```python
from build123d import *

# Parameters (mm, degrees)
SKETCH1_R           = 300
BOSS_EXTRUDE1_DEPTH = 8
SKETCH2_R           = 8
CUT_EXTRUDE1_DEPTH  = 425.339486732


with BuildPart() as part:
    # Sketch1 → Boss-Extrude1 (new body)
    with BuildSketch(Plane(origin=(0, 0, 0), x_dir=(1, 0, 0), z_dir=(0, 1, 0))):
        with Locations(Location((0, 0, 0), (0, 0, 270))):
            Circle(SKETCH1_R)
    extrude(amount=BOSS_EXTRUDE1_DEPTH)

    # Sketch2 → Cut-Extrude1 (cut, through all)
    with BuildSketch(Plane.XZ):
        with Locations(Location((0, 60, 0), (0, 0, 270))):
            Circle(SKETCH2_R)
        with Locations(Location((30, 51.961524227, 0), (0, 0, 270))):
            Circle(SKETCH2_R)
        with Locations(Location((51.961524227, 30, 0), (0, 0, 270))):
            Circle(SKETCH2_R)
        with Locations(Location((60, 0, 0), (0, 0, 270))):
            Circle(SKETCH2_R)
        with Locations(Location((51.961524227, -30, 0), (0, 0, 270))):
            Circle(SKETCH2_R)
        with Locations(Location((30, -51.961524227, 0), (0, 0, 270))):
            Circle(SKETCH2_R)
        with Locations(Location((0, -60, 0), (0, 0, 270))):
            Circle(SKETCH2_R)
        with Locations(Location((-30, -51.961524227, 0), (0, 0, 270))):
            Circle(SKETCH2_R)
        with Locations(Location((-51.961524227, -30, 0), (0, 0, 270))):
            Circle(SKETCH2_R)
        with Locations(Location((-60, 0, 0), (0, 0, 270))):
            Circle(SKETCH2_R)
        with Locations(Location((-51.961524227, 30, 0), (0, 0, 270))):
            Circle(SKETCH2_R)
        with Locations(Location((-30, 51.961524227, 0), (0, 0, 270))):
            Circle(SKETCH2_R)
    extrude(amount=-CUT_EXTRUDE1_DEPTH, mode=Mode.SUBTRACT)


solid = part.part
```
Read the model definition and answer for the solid it produces. Units are mm, in the model's axes. Coordinates: 2 decimals unless noted, no trailing zeros. Loops run counter-clockwise (first coordinate to the right, second up) from the corner with the lowest first, then second, coordinate; pieces in that order, holes last. Notation, with made-up numbers: (-29.5, 69.25) - (2.5, 69.25) arc R13 cw to (2.5, 82.25) - close; hole circle Ø3 at (-30.5, 7). An arc over 180 degrees is marked (long way). Answer in a Markdown table with one row per item.
1. Find section B-B, the plane z = 0. Write down the section's boundary in (x, y).
Conclusion:
| item | result |
|---|---|
| outline | (-300, 0) - (-68, 0) - (-68, 8) - (-300, 8) - close; (-52, 0) - (52, 0) - (52, 8) - (-52, 8) - close; (68, 0) - (300, 0) - (300, 8) - (68, 8) - close |
2. Find section D-D, the plane z = 240. Write down the section's boundary in (x, y).
Conclusion:
| item | result |
|---|---|
| outline | (-180, 0) - (180, 0) - (180, 8) - (-180, 8) - close |
3. Determine the mould class of faces 1 (the face through (-182.545, 3.944, -238.07)), 2 (the face through (4, 8, -4)), 3 (the face through (32.4, 3.94, 44.33)) for opening direction X: +X half, -X half, draft (parallel to the pull), parting line (faces both ways), or undercut.
Conclusion:
| item | result |
|---|---|
| face 1 | parting line |
| face 2 | draft |
| face 3 | undercut |
4. Straight lines are drawn through the part: line 1 (X direction, y = 4.25, z = 0); line 2 (Z direction, x = 45.5, y = 3.75); line 3 (Z direction, x = 6.5, y = 1.75). For each, find the intervals that lie inside material, in ascending order.
Conclusion:
| item | result |
|---|---|
| line 1 | x = -300 to -68, -52 to 52, 68 to 300 |
| line 2 | z = -296.53 to -34.72, -25.28 to 25.28, 34.72 to 296.53 |
| line 3 | z = -299.93 to -64.66, -55.34 to 55.34, 64.66 to 299.93 |
5. Given pin 1 (9.5 mm diameter, centred on x = -30, z = 51.96, fed in from +Y); pin 2 (3 mm diameter, centred on y = 2.5, z = -112.5, fed in from +X); pin 3 (4 mm diameter, centred on y = 2.5, z = -212.5, fed in from +X); pin 4 (4 mm diameter, centred on x = 142.5, y = 7, fed in from -Z), each flat-ended and moving along its own axis, determine where each tip first touches the part or whether it passes through.
Conclusion:
| item | result |
|---|---|
| pin 1 | passes through |
| pin 2 | stops at x = 278.71 |
| pin 3 | stops at x = 213.75 |
| pin 4 | stops at z = -265.07 |
6. Find section C-C, the plane y = 1.5. Count the separate pieces of the cut face and the enclosed holes in it, then the cut area to 3 significant figures.
Conclusion:
| item | result |
|---|---|
| separate pieces | 1 |
| enclosed holes | 12 |
| area | 280,000 mm² |
7. Find section A-A, the plane x = 0. Write down the section's boundary in (y, z).
Conclusion:
| item | result |
|---|---|
| outline | (0, -300) - (8, -300) - (8, -68) - (0, -68) - close; (0, -52) - (8, -52) - (8, 52) - (0, 52) - close; (0, 68) - (8, 68) - (8, 300) - (0, 300) - close |
